The listing builds one solid part. Answer for the finished solid, in the listing's coordinates (mm). Face numbers are marked on the shaded views. A direction names the side the tool comes from. Coordinates: 2 decimals unless noted, no trailing zeros. Loops run counter-clockwise (first coordinate to the right, second up) from the corner with the lowest first, then second, coordinate; pieces in that order, holes last. Notation, with made-up numbers: M 31,17.25 L 78,17.25 A29 ccw 78,40.25 Z; hole C -32,71 d4. An arc over 180 degrees is marked long. Answer as a JSON object with one key per item and string values. Group by question number.
1. A cutting plane is placed at A-A on y = 3.15. Give the vertices of the cut face in (x, z).
2. A cutting plane is placed at C-C on y = 0.65. Give the vertices of the cut face in (x, z), and give its area (3 significant figures).
3. Straight lines are drawn through the part: L1, parallel to Z at x = 16.25, y = 2.85; L2, parallel to X at y = 0.8, z = -10.5. For each, find the intervals that lie inside material, in ascending order.
4. For the marked faces 1, 2 and 3, determine the directions among +Z, -Z, +X, -X, +Y, -Y from which every point of the face is accessible in a straight line to the end or side of a thin tool.
5. Given pin 1 (1.5 mm diameter, centred on x = 11.5, y = 2.5, fed in from -Z), flat-ended and moving along its own axis, determine where the tip first touches the part or whether it passes through.
6. A cutting plane is placed at B-B on x = 10.5. Give the vertices of the cut face in (y, z), and give its area (3 significant figures).
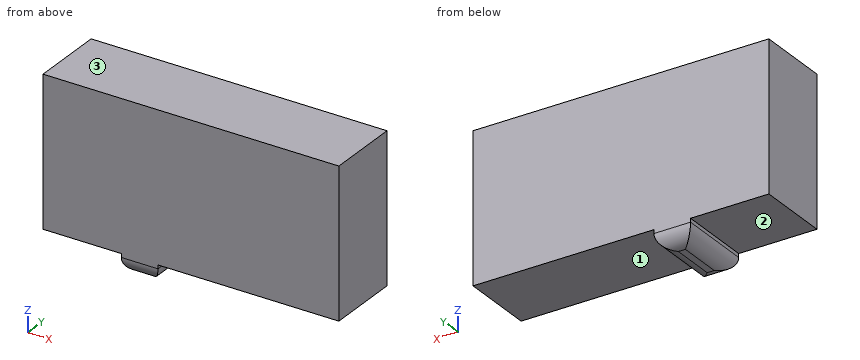
from build123d import *

# Parameters (mm, degrees)
SKETCH1_W           = 20.32
SKETCH1_H           = 10.16
BOSS_EXTRUDE1_DEPTH = 5.08
SKETCH3_W           = 2.516713444
SKETCH3_H           = 5.08
BOSS_EXTRUDE2_DEPTH = 1.27
FILLET1_R           = 1.016


with BuildPart() as part:
    # Sketch1 → Boss-Extrude1 (new body)
    with BuildSketch(Plane(origin=(0, 0, 0), x_dir=(1, 0, 0), z_dir=(0, 1, 0))):
        with Locations((10.16, 5.08)):
            Rectangle(SKETCH1_W, SKETCH1_H)
    extrude(amount=BOSS_EXTRUDE1_DEPTH)

    # Sketch3 → Boss-Extrude2 (add)
    with BuildSketch(Plane(origin=(0, 0, -10.16), x_dir=(-1, 0, 0), z_dir=(0, 0, -1))):
        with Locations((-6.637688848, 2.54)):
            Rectangle(SKETCH3_W, SKETCH3_H)
    extrude(amount=BOSS_EXTRUDE2_DEPTH)

    # Fillet1
    fillet1_edges = [part.edges().sort_by_distance(p)[0] for p in [
        (6.637688848, 0, -11.43),
        (5.379332126, 2.54, -11.43),
        (6.637688848, 5.08, -11.43),
        (7.89604557, 2.54, -11.43),
    ]]
    fillet(fillet1_edges, radius=FILLET1_R)


solid = part.part
From the geometry:
{
 "1": {"outline": "M 0,-10.16 L 5.38,-10.16 L 5.38,-10.41 A1.02 ccw 6.4,-11.43 L 6.88,-11.43 A1.02 ccw 7.9,-10.41 L 7.9,-10.16 L 20.32,-10.16 L 20.32,0 L 0,0 Z"},
 "2": {"outline": "M 0,-10.16 L 5.38,-10.16 L 5.38,-10.41 A1.02 ccw 6.03,-11.36 L 7.25,-11.36 A1.02 ccw 7.9,-10.41 L 7.9,-10.16 L 20.32,-10.16 L 20.32,0 L 0,0 Z", "area": "209 mm²"},
 "3": {"L1": "z = -10.16 to 0", "L2": "x = 5.38 to 7.89"},
 "4": {"face 1": "-Z, +X, +Y, -Y", "face 2": "-Z, -X, +Y, -Y", "face 3": "+Z, +X, -X, +Y, -Y"},
 "5": {"pin 1": "stops at z = -10.16"},
 "6": {"outline": "M 0,-10.16 L 5.08,-10.16 L 5.08,0 L 0,0 Z", "area": "51.6 mm²"}
}
